```python
from build123d import *

# Parameters (mm, degrees)
F1_DEPTH = 6
F3_DEPTH = 6
F5_DEPTH = 6


# Not quite as in the source:
# - a feature names something its author has since deleted; it is built from what else it names


with BuildPart() as f1:
    # F0 (on Top) → F1 (new body)
    with BuildSketch(Plane.XY):
        with BuildLine():
            Line((33, 13.8434663415), (-31, 13.8434663415))
            Line((-31, 13.8434663415), (-31, -11.1565336585))
            Line((-31, -11.1565336585), (33, -11.1565336585))
            Line((33, -11.1565336585), (33, -5.1422468387))
            Line((33, -5.1422468387), (13, -5.1422468387))
            ThreePointArc((13, -5.1422468387), (6.5, 1.3577531613), (13, 7.8577531613))
            Line((13, 7.8577531613), (33, 7.8577531613))
            Line((33, 7.8577531613), (33, 13.8434663415))
        make_face()
    extrude(amount=F1_DEPTH)

    # F2 (on face) → F3 (join)
    with BuildSketch(Plane(origin=(-31, 0, 0), x_dir=(0, -1, 0), z_dir=(-1, 0, 0))):
        with BuildLine():
            Line((-13.8434663415, 0), (11.1565336585, 0))
            Line((11.1565336585, 0), (11.1565336585, 15.6810280987))
            ThreePointArc((11.1565336585, 15.6810280987), (-1.3434663415, 4.3280202761), (-13.8434663415, 15.6810280987))
            Line((-13.8434663415, 15.6810280987), (-13.8434663415, 0))
        make_face()
        with BuildLine():
            ThreePointArc((-13.8434663415, 15.6810280987), (-1.3434663415, 4.3280202761), (11.1565336585, 15.6810280987))
            Line((11.1565336585, 15.6810280987), (11.1565336585, 18))
            Line((11.1565336585, 18), (5.0603540757, 18))
            ThreePointArc((5.0603540757, 18), (5.1324441239, 17.4450522775), (5.1565336585, 16.8859604746))
            ThreePointArc((5.1565336585, 16.8859604746), (-1.9025581444, 10.4100500092), (-7.7472867587, 18))
            Line((-7.7472867587, 18), (-13.8434663415, 18))
            Line((-13.8434663415, 18), (-13.8434663415, 15.6810280987))
        make_face()
        with BuildLine():
            Line((11.1565336585, 18), (11.1565336585, 15.6810280987))
            ThreePointArc((11.1565336585, 15.6810280987), (11.1999804438, 16.2827981629), (11.2144738571, 16.8859604746))
            ThreePointArc((11.2144738571, 16.8859604746), (-1.9466286532, 29.4294072599), (-13.8434663415, 15.6810280987))
            Line((-13.8434663415, 15.6810280987), (-13.8434663415, 18))
            Line((-13.8434663415, 18), (-7.7472867587, 18))
            ThreePointArc((-7.7472867587, 18), (-1.3434663415, 23.3859604746), (5.0603540757, 18))
            Line((5.0603540757, 18), (11.1565336585, 18))
        make_face()
    extrude(amount=F3_DEPTH)

    # F4 (on face) → F5 (join)
    with BuildSketch(Plane(origin=(0, 13.8434663415, 0), x_dir=(-1, 0, 0), z_dir=(0, 1, 0))):
        with BuildLine():
            Line((36.8821393698, 6), (11.8821393698, 6))
            Line((11.8821393698, 6), (11.8821393698, -10.7988112149))
            ThreePointArc((11.8821393698, -10.7988112149), (24.3821393698, 0.5575815545), (36.8821393698, -10.7988112149))
            Line((36.8821393698, -10.7988112149), (36.8821393698, 6))
        make_face()
        with BuildLine():
            ThreePointArc((36.8821393698, -10.7988112149), (24.3821393698, 0.5575815545), (11.8821393698, -10.7988112149))
            Line((11.8821393698, -10.7988112149), (11.8821393698, -12))
            Line((11.8821393698, -12), (17.8821393698, -12))
            ThreePointArc((17.8821393698, -12), (24.3821393698, -5.5), (30.8821393698, -12))
            Line((30.8821393698, -12), (36.8821393698, -12))
            Line((36.8821393698, -12), (36.8821393698, -10.7988112149))
        make_face()
        with BuildLine():
            Line((11.8821393698, -12), (11.8821393698, -10.7988112149))
            ThreePointArc((11.8821393698, -10.7988112149), (23.7808552995, -24.5431779053), (36.9397209243, -12))
            ThreePointArc((36.9397209243, -12), (36.9253172752, -11.3987159297), (36.8821393698, -10.7988112149))
            Line((36.8821393698, -10.7988112149), (36.8821393698, -12))
            Line((36.8821393698, -12), (30.8821393698, -12))
            ThreePointArc((30.8821393698, -12), (24.3821393698, -18.5), (17.8821393698, -12))
            Line((17.8821393698, -12), (11.8821393698, -12))
        make_face()
    extrude(amount=-F5_DEPTH)


solid = f1.part
```
Geometry check sheet. Reference: the model listing, model coordinates, mm. A direction names the side the tool comes from. Round coordinates to 2 decimals unless told otherwise and drop trailing zeros. Loops run counter-clockwise (first coordinate to the right, second up) from the corner with the lowest first, then second, coordinate; pieces in that order, holes last. Notation, with made-up numbers: (-8.75, 73) - (11.25, 73) arc R10 ccw to (11.25, 88) - close; hole circle Ø4 at (70.5, 56). An arc over 180 degrees is marked (long way). Write each question's results on one line, items separated by ' | '. Start each with the question number.
Q1. Cross-section at D-D on x = -23. Enter the section's corners in (y, z), and give its area (3 significant figures).
Q2. Cross-section at B-B on y = -3. Enter the section's corners in (x, z).
Q3. Gauge pin test, flat ends, axial feed: P1, Ø1.8, axis at y = 9.5, z = -7, coming from the +X side; P2, Ø12.5, axis at x = -6, y = 7, coming from the +Z side; P3, Ø1.5, axis at x = 25.5, z = 5.5, coming from the -Y side; P4, Ø5, axis at y = 2.5, z = 11, coming from the -X side. Record the tip position at first contact, or that the pin passes through.
Q4. Release check for a two-part mould opening along Z. For faces 1 (the flat face through (-37, 2, 8)), 2 (the cylindrical face through (-17.89, 10.89, -12.29)), 3 (the flat face through (-7, 2, 6)) record: +Z half, -Z half, draft (parallel to the pull), parting line (faces both ways), or undercut.
Q5. Cross-section at C-C on z = 2.5. Enter the section's corners in (x, y), and give its area (3 significant figures).
Q6. Cross-section at A-A on x = 9. Enter the section's corners in (y, z), and give its area (3 significant figures).
Q7. Access from +Z, -Z, +X, -X, +Y, -Y to the whole of each face (thin tool, end or side, straight path). Record for faces 4 (the flat face through (-9.3, 13.843, 0.3)), 5 (the flat face through (-2, -11.157, 4)), 6 (the flat face through (-31, 2, 10)), 7 (the flat face through (23, -5.142, 3)), 8 (the flat face through (-36.882, 11, -5)).
Q8. Thickness scan on line 1 (X direction, y = 10.3, z = -12); line 2 (Z direction, x = -30, y = 1.25); line 3 (X direction, y = 11.25, z = -5). Record the ranges inside material, lowest first. Write a range as [from, to].
Answers below:
1) outline: (-11.16, 0) - (7.84, 0) - (7.84, -5.65) - (13.84, -5.65) - (13.84, 6) - (-11.16, 6) - close; (7.84, -24.48) - (13.84, -24.48) - (13.84, -18.35) - (7.84, -18.35) - close | area: 221 mm²
2) outline: (-37, 0) - (8.18, 0) - (8.18, 6) - (-31, 6) - (-31, 12.05) - (-37, 12.05) - close; (-37, 21.72) - (-31, 21.72) - (-31, 28.67) - (-37, 28.67) - close
3) P1: stops at x = -11.88 | P2: stops at z = 6 | P3: stops at y = -11.16 | P4: stops at x = -37
4) face 1: draft | face 2: undercut | face 3: +Z half
5) outline: (-37, -11.16) - (33, -11.16) - (33, -5.14) - (13, -5.14) arc R6.5 cw to (13, 7.86) - (33, 7.86) - (33, 13.84) - (-37, 13.84) - close | area: 1,420 mm²
6) outline: (-11.16, 0) - (-3.77, 0) - (-3.77, 6) - (-11.16, 6) - close; (6.48, 0) - (13.84, 0) - (13.84, 6) - (6.48, 6) - close | area: 88.5 mm²
7) face 4: -Z, +X, -X, +Y | face 5: -Z, +X, -X, -Y | face 6: +Z, +X, +Y, -Y | face 7: +Z, -Z, +X | face 8: -X, +Y, -Y
8) line 1: x = [-36.94, -30.88], [-17.88, -11.82] | line 2: z = [0, 6] | line 3: x = [-36.88, -11.88]
